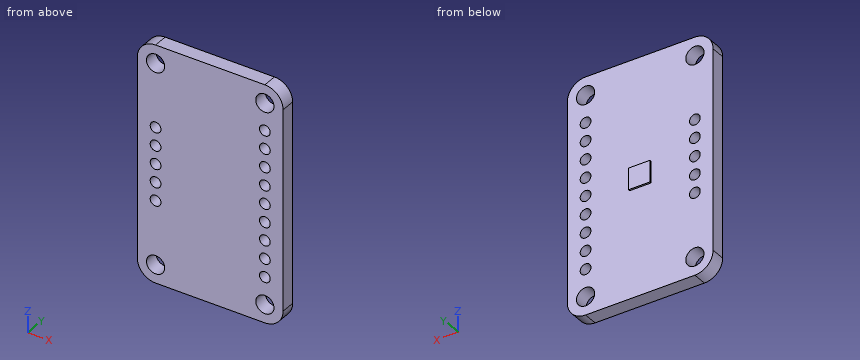
Autodesk Inventor part; units mm, degrees
ref_plane "YZ Plane" through (0, 0, 0) normal (1, 0, 0) x (0, 1, 0)
ref_plane "XZ Plane" through (0, 0, 0) normal (0, 1, 0) x (-1, 0, 0)
ref_plane "XY Plane" through (0, 0, 0) normal (0, 0, 1) x (1, 0, 0)
sketch "Sketch1" plane through (0, 0, 0) normal (0, 1, 0) x (-1, 0, 0)
  line L0 (0, 0) -> (10.16, 0)
  line L1 (10.16, 0) -> (10.16, -13.97)
  line L2 (10.16, 0) -> (10.16, 13.97)
  line L3 (10.16, 0) -> (24.13, 0) construction
  line L4 (0, 0) -> (-10.16, 0)
  line L5 (0, 0) -> (10.16, 0) construction
  line L6 (-10.16, 0) -> (-10.16, -13.97)
  line L7 (-10.16, 0) -> (-10.16, 13.97)
  line L8 (-10.16, 13.97) -> (-7.62, 13.97)
  arc A0 (-7.62, 16.51) -> (-10.16, 13.97) centre (-7.62, 13.97) ccw
  line L9 (-7.62, 13.97) -> (-7.62, 16.51) construction
  line L10 (-7.62, 13.97) -> (-10.16, 13.97) construction
  line L11 (0, 0) -> (0, -1)
  line L12 (10.16, 13.97) -> (7.62, 13.97)
  line L13 (10.16, 13.97) -> (12.7, 13.97) construction
  arc A1 (10.16, 13.97) -> (7.62, 16.51) centre (7.62, 13.97) ccw
  line L14 (7.62, 13.97) -> (7.62, 16.51) construction
  line L15 (7.62, 13.97) -> (10.16, 13.97) construction
  line L16 (-7.62, 16.51) -> (7.62, 16.51)
  line L17 (10.16, -13.97) -> (7.62, -13.97)
  line L18 (10.16, -13.97) -> (12.7, -13.97) construction
  line L19 (-10.16, -13.97) -> (-7.62, -13.97)
  arc A2 (7.62, -16.51) -> (10.16, -13.97) centre (7.62, -13.97) ccw
  arc A3 (-10.16, -13.97) -> (-7.62, -16.51) centre (-7.62, -13.97) ccw
  line L20 (-7.62, -16.51) -> (7.62, -16.51)
  dimension "d0" = 10.16
  dimension "d1" = 13.97
  dimension "d2" = 13.97
  dimension "d3" = 90
  dimension "d4" = 10.16
  dimension "d5" = 180
  dimension "d6" = 13.97
  dimension "d7" = 13.97
  dimension "d8" = 2.54
  dimension "d9" = 90
  dimension "d11" = 1
  dimension "d12" = 2.54
  dimension "d13" = 180
  dimension "d14" = 90
  dimension "d15" = 2.54
  dimension "d16" = 180
  dimension "d17" = 2.54
  dimension "d18" = 15.24
extrude "Extrusion1" add sketch "Sketch1" along normal blind 2
sketch "Sketch2" plane through (0, 2, 0) normal (0, 1, 0) x (1, 0, 0)
  line L0 (0, 0) -> (7.62, 0)
  line L1 (0, 0) -> (-7.62, 0)
  circle A0 centre (7.62, 0) radius 0.75
  line L2 (0, 0) -> (0, 1)
  circle A1 centre (7.62, 2.54) radius 0.75
  circle A2 centre (7.62, 5.08) radius 0.75
  circle A3 centre (7.62, 7.62) radius 0.75
  circle A4 centre (7.62, 10.16) radius 0.75
  circle A5 centre (7.62, -2.54) radius 0.75
  circle A6 centre (7.62, 0) radius 0.75
  circle A7 centre (7.62, 2.54) radius 0.75
  circle A8 centre (7.62, 5.08) radius 0.75
  circle A9 centre (7.62, 7.62) radius 0.75
  circle A10 centre (7.62, -5.08) radius 0.75
  circle A11 centre (7.62, -2.54) radius 0.75
  circle A12 centre (7.62, 0) radius 0.75
  circle A13 centre (7.62, 2.54) radius 0.75
  circle A14 centre (7.62, 5.08) radius 0.75
  circle A15 centre (7.62, -7.62) radius 0.75
  circle A16 centre (7.62, -5.08) radius 0.75
  circle A17 centre (7.62, -2.54) radius 0.75
  circle A18 centre (7.62, 0) radius 0.75
  circle A19 centre (7.62, 2.54) radius 0.75
  circle A20 centre (7.62, -10.16) radius 0.75
  circle A21 centre (7.62, -7.62) radius 0.75
  circle A22 centre (7.62, -5.08) radius 0.75
  circle A23 centre (7.62, -2.54) radius 0.75
  circle A24 centre (7.62, 0) radius 0.75
  circle A25 centre (-7.62, 0) radius 0.75
  circle A26 centre (-7.62, 2.54) radius 0.75
  circle A27 centre (-7.62, 5.08) radius 0.75
  circle A28 centre (-7.62, -2.54) radius 0.75
  circle A29 centre (-7.62, 0) radius 0.75
  circle A30 centre (-7.62, 2.54) radius 0.75
  circle A31 centre (-7.62, -5.08) radius 0.75
  circle A32 centre (-7.62, -2.54) radius 0.75
  circle A33 centre (-7.62, 0) radius 0.75
  dimension "d21" = 7.62
  dimension "d22" = 7.62
  dimension "d23" = 1.5
  dimension "d24" = 1
  dimension "d27" = 2.54
  dimension "d30" = 2.54
  dimension "d33" = 1.5
  dimension "d36" = 2.54
  dimension "d39" = 2.54
extrude "Extrusion2" cut sketch "Sketch2" against normal blind 2
sketch "Sketch3" plane through (0, 2, 0) normal (0, 1, 0) x (1, 0, 0)
  line L0 (1.5, -1.5) -> (-1.5, -1.5)
  line L1 (-1.5, -1.5) -> (-1.5, 1.5)
  line L2 (-1.5, 1.5) -> (1.5, 1.5)
  line L3 (1.5, 1.5) -> (1.5, -1.5)
  line L4 (1.5, -1.5) -> (-1.5, 1.5) construction
  line L5 (-1.5, -1.5) -> (1.5, 1.5) construction
  point P0 (0, 0)
  dimension "d44" = 3
  dimension "d45" = 3
extrude "Extrusion3" add sketch "Sketch3" along normal blind 0.25
sketch "Sketch4" plane through (0, 2, 0) normal (0, 1, 0) x (1, 0, 0)
  arc A0 (7.62, -16.51) -> (10.16, -13.97) centre (7.62, -13.97) ccw
  circle A1 centre (7.62, -13.97) radius 1.27
  line L0 (1.5, -1.5) -> (1.5, 1.5)
  line L1 (1.5, -1.5) -> (1.5, 1.5)
  line L2 (-1.5, 1.5) -> (-1.5, -1.5)
  line L3 (1.5, 1.5) -> (-1.5, 1.5)
  circle A2 centre (7.62, 13.97) radius 1.27
  circle A3 centre (-7.62, -13.97) radius 1.27
  circle A4 centre (-7.62, 13.97) radius 1.27
  point P0 (0, 0)
  dimension "d48" = 2.54
  dimension "d51" = 27.94
  dimension "d54" = 15.24
extrude "Extrusion4" cut sketch "Sketch4" against normal blind 2
properties part number "LSM9DS1"
Can you work these out from the model? Positions are in its coordinate system, mm. Round coordinates to 2 decimals unless told otherwise and drop trailing zeros. Loops run counter-clockwise (first coordinate to the right, second up) from the corner with the lowest first, then second, coordinate; pieces in that order, holes last. Notation, with made-up numbers: (29, 44.25) - (76, 44.25) arc R27 ccw to (76, 66.25) - close; hole circle Ø9 at (-7, -27.5). An arc over 180 degrees is marked (long way). Use CSV: the item, a comma, the result in double quotes. Start each with the question number.
1) For pin 1 Ø1.4 at (x, z) = (7.62, -10.16) entering from -Y; pin 2 Ø6 at (x, z) = (-4.5, -4) entering from +Y, each with a flat end and sliding along its axis, tell me the tip position at first contact or that it passes through.
2) Please list where these lines run through material, in increasing order: probe 1 along X at (y, z) = (1.05, 0); probe 2 along Y at (x, z) = (1.5, -8.5); probe 3 along X at (y, z) = (1.7, 10). Write a range as [from, to].
3) If we section it at C-C on z = 8: Write out the boundary of the cut face in (x, y).
4) If we section it at D-D on z = -10.16: Write out the boundary of the cut face in (x, y), plus the area to 3 significant figures.
5) If we section it at B-B on y = 0.8: Count the separate pieces of the cut face and the enclosed holes in it, plus the area to 3 significant figures.
6) If we section it at A-A on z = 0: Write out the boundary of the cut face in (x, y).
Geometry results:
1,pin 1,"passes through"
1,pin 2,"stops at y = 2"
2,probe 1,"x = [-10.16, -8.37], [-6.87, 6.87], [8.37, 10.16]"
2,probe 2,"y = [0, 2]"
2,probe 3,"x = [-10.16, 6.89], [8.35, 10.16]"
3,outline,"(-10.16, 0) - (6.97, 0) - (6.97, 2) - (-10.16, 2) - close; (8.27, 0) - (10.16, 0) - (10.16, 2) - (8.27, 2) - close"
4,outline,"(-10.16, 0) - (6.87, 0) - (6.87, 2) - (-10.16, 2) - close; (8.37, 0) - (10.16, 0) - (10.16, 2) - (8.37, 2) - close"
4,area,"37.6 mm2"
5,separate pieces,"1"
5,enclosed holes,"18"
5,area,"620 mm2"
6,outline,"(-10.16, 0) - (-8.37, 0) - (-8.37, 2) - (-10.16, 2) - close; (-6.87, 0) - (6.87, 0) - (6.87, 2) - (1.5, 2) - (1.5, 2.25) - (-1.5, 2.25) - (-1.5, 2) - (-6.87, 2) - close; (8.37, 0) - (10.16, 0) - (10.16, 2) - (8.37, 2) - close"
